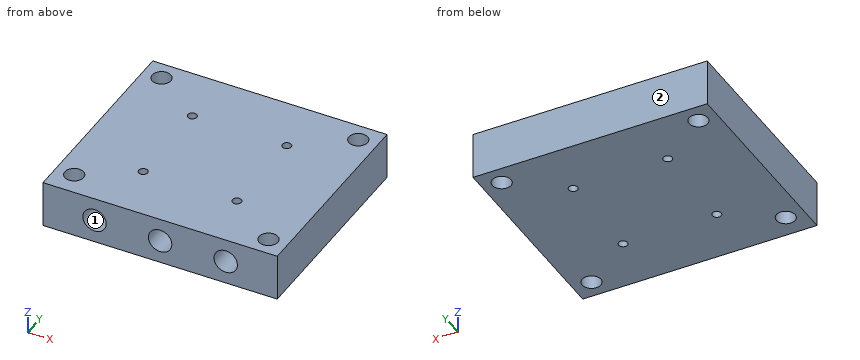
from build123d import *

# Parameters (mm, degrees)
SKETCH2_W                          = 5
SKETCH2_H                          = 22
BOSS_EXTRUDE1_DEPTH                = 25
TAP_DRILL_FOR_M2_5X0_45_TAP1_D     = 2.5
TAP_DRILL_FOR_M2_5X0_45_TAP1_DEPTH = 5
TAP_DRILL_FOR_M1_2X0_25_TAP1_D     = 0.95
TAP_DRILL_FOR_M2X0_4_TAP1_D        = 2


with BuildPart() as part:
    # Sketch2 → Boss-Extrude1 (new body)
    with BuildSketch(Plane(origin=(0, 0, 0), x_dir=(0, 0, -1), z_dir=(1, 0, 0))):
        with Locations((2.5, 5)):
            Rectangle(SKETCH2_W, SKETCH2_H)
    extrude(amount=BOSS_EXTRUDE1_DEPTH)

    # Tap Drill for M2.5x0.45 Tap1
    with Locations(Plane(origin=(0, -6, 0), x_dir=(-1, 0, 0), z_dir=(0, -1, 0))):
        with Locations((-19.5, 2.5), (-12.5, 2.5), (-5.5, 2.5)):
            Hole(TAP_DRILL_FOR_M2_5X0_45_TAP1_D / 2, depth=TAP_DRILL_FOR_M2_5X0_45_TAP1_DEPTH)

    # Tap Drill for M1.2x0.25 Tap1 (through all)
    with Locations(Plane(origin=(0, 0, -5), x_dir=(-1, 0, 0), z_dir=(0, 0, -1))):
        with Locations((-17.5, 10), (-7.413132908, 10), (-17.5, 0), (-7.5, 0)):
            Hole(TAP_DRILL_FOR_M1_2X0_25_TAP1_D / 2)

    # Tap Drill for M2x0.4 Tap1 (through all)
    with Locations(Plane.XY):
        with Locations((2, 14), (2, -3.5), (23, -4), (23, 14)):
            Hole(TAP_DRILL_FOR_M2X0_4_TAP1_D / 2)


solid = part.part
Work out the finished part from the listing and answer in its coordinate system (mm). Face numbers are marked on the shaded views. A direction names the side the tool comes from. Give positions to 0.01 mm unless a question says otherwise; leave off trailing zeros. Order: outer loops, then holes, each group sorted by start corner. A loop starts at its lowest first (then second) coordinate and runs counter-clockwise, first axis right, second up. Notation, with made-up numbers: M 44,24 L 82,24 A22 ccw 82,40 Z; hole C 83.5,-33 d11. An arc over 180 degrees is marked long. Return JSON: item names as keys, results as strings.
Q1. Which of the six approach directions +Z, -Z, +X, -X, +Y, -Y give full straight-line access (tool end or side, diameter ignored) to the marked faces 1 and 2?
Answer below:
{"face 1": "-Y", "face 2": "+Z, -Z, +X, -X, +Y"}
Q2. Find section A-A, the plane y = -3.5. Write down the section's boundary in (x, z), and give its area (3 significant figures).
Answer below:
{"outline": "M 0,-5 L 1,-5 L 1,0 L 0,0 Z; M 3,-5 L 22.13,-5 L 22.13,0 L 3,0 Z; M 23.87,-5 L 25,-5 L 25,0 L 23.87,0 Z; hole C 5.5,-2.5 d2.5; hole C 12.5,-2.5 d2.5; hole C 19.5,-2.5 d2.5", "area": "91.6 mm^2"}
Q3. Find section D-D, the plane z = -2.1. State how many separate pieces and enclosed holes the cut face has, and give its area (3 significant figures).
Answer below:
{"separate pieces": "1", "enclosed holes": "8", "area": "499 mm^2"}
Q4. Find the intervals of material crossed by line 1 along Y through (x, z) = (17.5, -3.1) (3 decimals); line 2 along Y through (x, z) = (2, -3.75); line 3 along X through (y, z) = (-0.25, -1.1), in increasing order. Write a range as [from, to].
Answer below:
{"line 1": "y = [-6, -0.475], [0.475, 9.525], [10.475, 16]", "line 2": "y = [-6, -4.5], [-2.5, 13], [15, 16]", "line 3": "x = [0, 7.1], [7.9, 17.1], [17.9, 25]"}
Q5. This flat-tipped pin is pushed along its axis until it touches: pin 1 (1.5 mm diameter, centred on x = 12.5, z = -2.5, fed in from -Y). Where does it stop, or does it pass through?
Answer below:
{"pin 1": "stops at y = -1"}
Q6. Find section B-B, the plane x = 23. Write down the section's boundary in (y, z).
Answer below:
{"outline": "M -6,-5 L -5,-5 L -5,0 L -6,0 Z; M -3,-5 L 13,-5 L 13,0 L -3,0 Z; M 15,-5 L 16,-5 L 16,0 L 15,0 Z"}
Q7. Find section C-C, the plane y = 0. Write down the section's boundary in (x, z) (3 decimals), and give its area (4 significant figures).
Answer below:
{"outline": "M 0,-5 L 7.025,-5 L 7.025,0 L 0,0 Z; M 7.975,-5 L 17.025,-5 L 17.025,0 L 7.975,0 Z; M 17.975,-5 L 25,-5 L 25,0 L 17.975,0 Z", "area": "115.5 mm^2"}
